Check sheet for the modelled part. Datum: model origin and axes. Units: mm. A direction names the side the tool comes from. Coordinates: 2 decimals unless noted, no trailing zeros. Loops run counter-clockwise (first coordinate to the right, second up) from the corner with the lowest first, then second, coordinate; pieces in that order, holes last.
```python
from build123d import *

# Parameters (mm, degrees)
SKETCH1_W                      = 100
SKETCH1_H                      = 50
BOSS_EXTRUDE1_DEPTH            = 10
M6_CLEARANCE_HOLE1_D           = 6.6
M6_CLEARANCE_HOLE1_CSINK_D     = 6.65
M6_CLEARANCE_HOLE1_CSINK_ANGLE = 100
SKETCH4_W                      = 30
SKETCH4_H                      = 40
BOSS_EXTRUDE2_DEPTH            = 107.84
BOSS_EXTRUDE3_DEPTH            = 50
BOSS_EXTRUDE3_DEPTH_BACK       = 50
SKETCH6_W                      = 40
SKETCH6_H                      = 30
SKETCH7_W                      = 20
SKETCH7_H                      = 40
BOSS_EXTRUDE4_DEPTH            = 60
SKETCH8_R                      = 13
CUT_EXTRUDE3_DEPTH             = 206.553072465


with BuildPart() as part:
    # Sketch1 → Boss-Extrude1 (new body)
    with BuildSketch(Plane(origin=(0, 0, 0), x_dir=(1, 0, 0), z_dir=(0, 1, 0))):
        Rectangle(SKETCH1_W, SKETCH1_H)
    extrude(amount=BOSS_EXTRUDE1_DEPTH)

    # M6 Clearance Hole1 (through all)
    with Locations(Plane(origin=(0, 10, 0), x_dir=(1, 0, 0), z_dir=(0, 1, 0))):
        with Locations((-40, 15), (40, 15), (-40, -15), (40, -15)):
            CounterSinkHole(M6_CLEARANCE_HOLE1_D / 2, M6_CLEARANCE_HOLE1_CSINK_D / 2, counter_sink_angle=M6_CLEARANCE_HOLE1_CSINK_ANGLE)

    # Sketch4 → Boss-Extrude2 (add)
    with BuildSketch(Plane(origin=(0, 10, 0), x_dir=(1, 0, 0), z_dir=(0, 1, 0))):
        Rectangle(SKETCH4_W, SKETCH4_H)
    extrude(amount=BOSS_EXTRUDE2_DEPTH)

    # Sketch6 → Boss-Extrude3 (add, two sides: drawn at the far end of the back side and taken through both)
    with BuildSketch(Plane(origin=(0, 0, 0), x_dir=(0, 0, -1), z_dir=(1, 0, 0)).offset(-BOSS_EXTRUDE3_DEPTH_BACK)):
        with Locations((0, 102.84)):
            Rectangle(SKETCH6_W, SKETCH6_H)
    extrude(amount=BOSS_EXTRUDE3_DEPTH + BOSS_EXTRUDE3_DEPTH_BACK)

    # Sketch7 → Boss-Extrude4 (add)
    with BuildSketch(Plane(origin=(0, 117.84, 0), x_dir=(1, 0, 0), z_dir=(0, 1, 0))):
        with Locations((-40, 0)):
            Rectangle(SKETCH7_W, SKETCH7_H)
        with Locations((40, 0)):
            Rectangle(SKETCH7_W, SKETCH7_H)
    extrude(amount=BOSS_EXTRUDE4_DEPTH)

    # Sketch8 → Cut-Extrude3 (cut, through all)
    with BuildSketch(Plane.ZY.offset(50)):
        with Locations((0, 137.84)):
            Circle(SKETCH8_R)
    extrude(amount=-CUT_EXTRUDE3_DEPTH, mode=Mode.SUBTRACT)


solid = part.part
```
1) Section check D-D on y = 137.84. Enter the section's corners in (x, z), plus the area to 3 significant figures.
Answer sheet:
outline: (-50, -20) - (-30, -20) - (-30, -13) - (-50, -13) - close; (-50, 13) - (-30, 13) - (-30, 20) - (-50, 20) - close; (30, -20) - (50, -20) - (50, -13) - (30, -13) - close; (30, 13) - (50, 13) - (50, 20) - (30, 20) - close
area: 560 mm2
2) Scan lines: line 1 (Z direction, x = -40, y = 6.25); line 2 (X direction, y = 6, z = -15); line 3 (X direction, y = 134, z = 18.5). Record each from-to range of solid material in increasing order.
Answer sheet:
line 1: z = -25 to -18.3, -11.7 to 11.7, 18.3 to 25
line 2: x = -50 to -43.3, -36.7 to 36.7, 43.3 to 50
line 3: x = -50 to -30, 30 to 50
3) Mould release check, pull along Z, two halves, no side actions. Record for faces 6 (the cylindrical face through (-37.381, 4.92, 17.008)), 7 (the flat face through (32, 87.84, 0)), 8 (the flat face through (-1, 5, 25)): +Z half, -Z half, draft (parallel to the pull), parting line (faces both ways), or undercut.
Answer sheet:
face 6: undercut
face 7: draft
face 8: +Z half
4) Section check A-A on x = -33.5. Enter the section's corners in (y, z).
Answer sheet:
outline: (0, -25) - (10, -25) - (10, 25) - (0, 25) - close; (87.84, -20) - (177.84, -20) - (177.84, 20) - (87.84, 20) - close; hole circle Ø26 at (137.84, 0)
5) Depth check by flat-ended pin: pin 1 (3 mm diameter, centred on y = 24, z = -9.5, fed in from -X); pin 2 (8 mm diameter, centred on x = -33.5, z = 13, fed in from -Y); pin 3 (20 mm diameter, centred on x = 3.5, z = 4.5, fed in from +Y); pin 4 (20 mm diameter, centred on y = 49, z = 0, fed in from +X). Enter the tip coordinate at first touch or a pass-through.
Answer sheet:
pin 1: stops at x = -15
pin 2: stops at y = 0
pin 3: stops at y = 117.84
pin 4: stops at x = 15
6) Section check B-B on z = -15. Enter the section's corners in (x, y) (3 decimals), plus the area to 3 significant figures.
Answer sheet:
outline: (-50, 0) - (-43.3, 0) - (-43.3, 9.979) - (-43.325, 10) - (-50, 10) - close; (-50, 87.84) - (-15, 87.84) - (-15, 10) - (-36.675, 10) - (-36.7, 9.979) - (-36.7, 0) - (36.7, 0) - (36.7, 9.979) - (36.675, 10) - (15, 10) - (15, 87.84) - (50, 87.84) - (50, 177.84) - (30, 177.84) - (30, 117.84) - (-30, 117.84) - (-30, 177.84) - (-50, 177.84) - close; (43.3, 0) - (50, 0) - (50, 10) - (43.325, 10) - (43.3, 9.979) - close
area: 8,600 mm2
7) Set-up check for faces 1 (the flat face through (15, 48, 0)), 2 (the flat face through (-30, 154, 0)), 3 (the flat face through (-1, 93, -20)), 4 (the cylindrical face through (-37.381, 4.92, -12.992)), 5 (the flat face through (-15, 48, 0)): record each of +Z, -Z, +X, -X, +Y, -Y from which the full face is reachable in a straight line by a thin tool's end or side.
Answer sheet:
face 1: +Z, -Z, +X
face 2: +Z, -Z, +Y
face 3: -Z, +X, -X, +Y
face 4: -Y
face 5: +Z, -Z, -X
8) Section check C-C on x = 40. Enter the section's corners in (y, z) (3 decimals), plus the area to 3 significant figures.
Answer sheet:
outline: (0, -25) - (10, -25) - (10, -18.325) - (9.979, -18.3) - (0, -18.3) - close; (0, -11.7) - (9.979, -11.7) - (10, -11.675) - (10, 11.675) - (9.979, 11.7) - (0, 11.7) - close; (0, 18.3) - (9.979, 18.3) - (10, 18.325) - (10, 25) - (0, 25) - close; (87.84, -20) - (177.84, -20) - (177.84, 20) - (87.84, 20) - close; hole circle Ø26 at (137.84, 0)
area: 3,440 mm2
